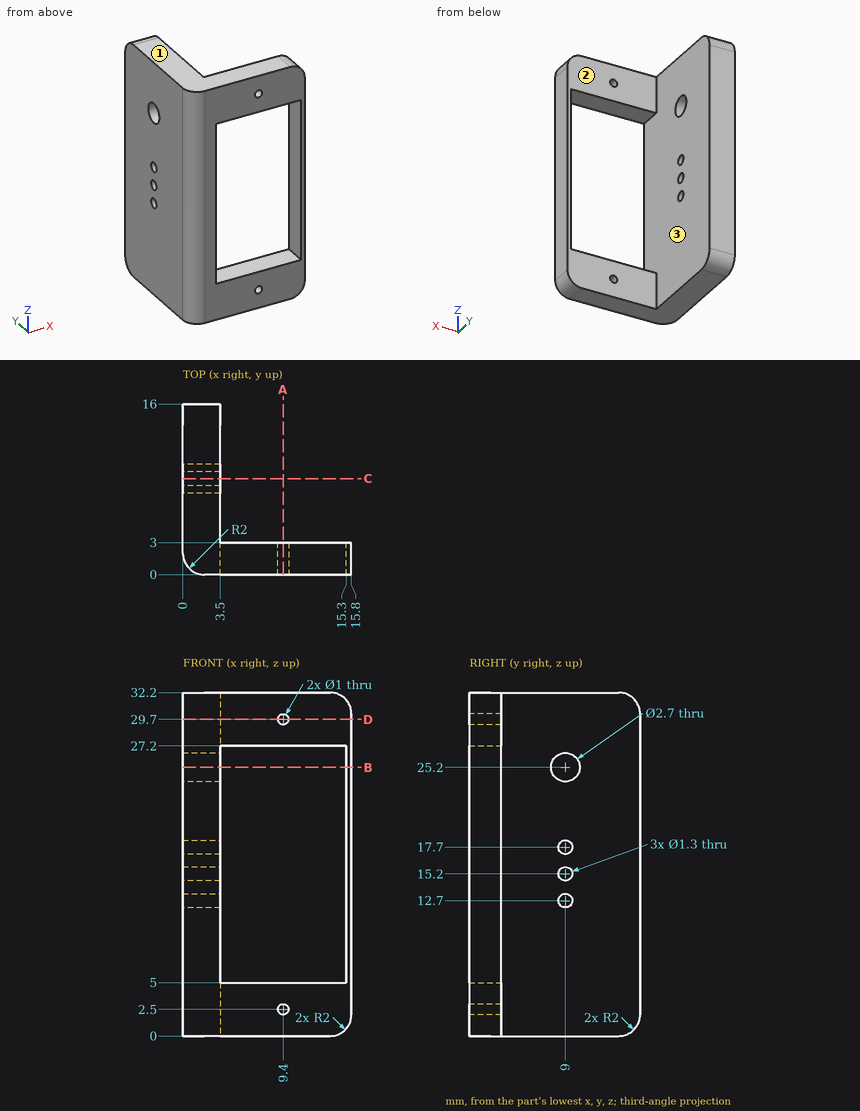
Answer from the drawing. Dimensions are ordinates in mm from the lowest x, y and z of the part. A direction names the side the tool comes from. Give positions to 0.01 mm unless a question says otherwise; leave off trailing zeros. Loops run counter-clockwise (first coordinate to the right, second up) from the corner with the lowest first, then second, coordinate; pieces in that order, holes last. Notation, with made-up numbers: M 26.5,-22 L 64.5,-22 A19 cw 64.5,0 Z; hole C 67,44.25 d6. An arc over 180 degrees is marked long. One line per item, written item: value.
Q1. A cutting plane is placed at B-B on z = 25.2. Determine the outline of the cut face in (x, y).
Working result:
outline: M 0,2 A2 ccw 2,0 L 3.5,0 L 3.5,7.65 L 0,7.65 Z; M 0,10.35 L 3.5,10.35 L 3.5,16 L 0,16 Z; M 15.3,0 L 15.8,0 L 15.8,3 L 15.3,3 Z
Q2. Flat-ended cylindrical pins translate along their axes: P1, Ø1.5, axis at y = 11, z = 19, coming from the +X side; P2, Ø3.5, axis at x = 11, y = 1.5, coming from the -Z side; P3, Ø6, axis at x = 9, z = 22, coming from the +Y side; P4, Ø1.5, axis at x = 12, z = 28, coming from the +Y side. Find the tip coordinate at first contact, or state that the pin passes through.
Working result:
P1: stops at x = 3.5
P2: stops at z = 0
P3: passes through
P4: stops at y = 3
Q3. For the marked faces 1, 2 and 3, determine the directions among +Z, -Z, +X, -X, +Y, -Y from which every point of the face is accessible in a straight line to the end or side of a thin tool.
Working result:
face 1: +Z, +X, -X, +Y, -Y
face 2: +Z, -Z, +X, +Y
face 3: +Y
Q4. A cutting plane is placed at A-A on x = 9.4. Determine the outline of the cut face in (y, z), then the cut area to 3 significant figures.
Working result:
outline: M 0,0 L 3,0 L 3,2 L 0,2 Z; M 0,3 L 3,3 L 3,5 L 0,5 Z; M 0,27.2 L 3,27.2 L 3,29.2 L 0,29.2 Z; M 0,30.2 L 3,30.2 L 3,32.2 L 0,32.2 Z
area: 24.0 mm^2
Q5. Find the intervals of material crossed by line 1 (Z direction, x = 6.5, y = 2.5); line 2 (X direction, y = 11.75, z = 4.5); line 3 (Y direction, x = 2.15, z = 17.7), in increasing order. Write a range as from..to.
Working result:
line 1: z = 0..5, 27.2..32.2
line 2: x = 0..3.5
line 3: y = 0..8.35, 9.65..16
Q6. A cutting plane is placed at C-C on y = 9. Determine the outline of the cut face in (x, z), then the cut area to 3 significant figures.
Working result:
outline: M 0,0 L 3.5,0 L 3.5,12.05 L 0,12.05 Z; M 0,13.35 L 3.5,13.35 L 3.5,14.55 L 0,14.55 Z; M 0,15.85 L 3.5,15.85 L 3.5,17.05 L 0,17.05 Z; M 0,18.35 L 3.5,18.35 L 3.5,23.85 L 0,23.85 Z; M 0,26.55 L 3.5,26.55 L 3.5,32.2 L 0,32.2 Z
area: 89.6 mm^2
Q7. A cutting plane is placed at D-D on z = 29.7. Determine the outline of the cut face in (x, y), then the cut area to 3 significant figures.
Working result:
outline: M 0,2 A2 ccw 2,0 L 8.9,0 L 8.9,3 L 3.5,3 L 3.5,16 L 0,16 Z; M 9.9,0 L 15.8,0 L 15.8,3 L 9.9,3 Z
area: 89.0 mm^2
